Verification items for the finished model (mm, model axes). Give positions to 0.01 mm unless a question says otherwise; leave off trailing zeros. Order: outer loops, then holes, each group sorted by start corner. A loop starts at its lowest first (then second) coordinate and runs counter-clockwise, first axis right, second up. Notation, with made-up numbers: (-23, 75) -> (3, 75) arc R14 ccw to (3, 86) -> close; hole circle Ø10 at (-13, 23.5). An arc over 180 degrees is marked (long way). Return JSON: item names as keys, results as strings. Group by question number.
(1) Release check for a two-part mould opening along Y. For faces 1 (the face through (16.31, 40.067, 57.291)), 2 (the face through (18, 38, 0)), 3 (the face through (18.13, 46.87, 55.71)) record: pulls with the +Y half, pulls with the -Y half, needs draft (parallel to the pull), parting line crosses it, or undercut.
(2) Thickness scan on line 1 along Y through (x, z) = (16.25, 99); line 2 along Y through (x, z) = (18.5, 8); line 3 along X through (y, z) = (39.75, 71.5). Record the ranges inside material, lowest first.
(3) Cross-section at A-A on z = 100.5. Enter the section's corners in (x, y).
(4) Depth check by flat-ended pin: pin 1 Ø4 at (y, z) = (33.5, 20) entering from -X; pin 2 Ø1.5 at (y, z) = (42.5, 31) entering from -X; pin 3 Ø5 at (x, y) = (17.5, 40.98) entering from -Z; pin 4 Ø4 at (x, z) = (14, 77) entering from +Y. Enter the tip coordinate at first touch or a pass-through.
from build123d import *

# Parameters (mm, degrees)
RESSALTO_EXTRUS_O1_DEPTH = 113
ESBO_O2_R                = 1.5
CORTE_EXTRUS_O1_DEPTH    = 113


with BuildPart() as part:
    # Esboço1 → Ressalto-extrusão1 (new body)
    with BuildSketch(Plane.XY):
        Polygon((11.5, 30.979337094), (21.5, 30.979337094), (21.5, 49.687624028), (21.161059666, 49.456664041), (19.066345307, 47.808952584), (17.161004874, 45.902414631), (15.486453, 43.765993321), (14.074906639, 41.431162512), (12.967287062, 38.97151993), (12.155978451, 36.372733292), (11.660337074, 33.660653998), align=None)
    extrude(amount=RESSALTO_EXTRUS_O1_DEPTH)

    # Esboço2 → Corte-extrusão1 (cut)
    with BuildSketch(Plane.XY.offset(113)):
        with Locations((17.5, 34.979337094)):
            Circle(ESBO_O2_R)
        with Locations((17.5, 40.979337094)):
            Circle(ESBO_O2_R)
    extrude(amount=-CORTE_EXTRUS_O1_DEPTH, mode=Mode.SUBTRACT)


solid = part.part
Verdict:
{
 "1": {"face 1": "undercut", "face 2": "needs draft", "face 3": "pulls with the +Y half"},
 "2": {"line 1": "30.98 to 34.15, 35.81 to 40.15, 41.81 to 44.74", "line 2": "30.98 to 33.86, 36.1 to 39.86, 42.1 to 47.24", "line 3": "13.32 to 16.64, 18.36 to 21.5"},
 "3": {"outline": "(11.5, 30.98) -> (21.5, 30.98) -> (21.5, 49.69) -> (21.16, 49.46) -> (19.07, 47.81) -> (17.16, 45.9) -> (15.49, 43.77) -> (14.07, 41.43) -> (12.97, 38.97) -> (12.16, 36.37) -> (11.66, 33.66) -> close; hole circle Ø3 at (17.5, 34.98); hole circle Ø3 at (17.5, 40.98)"},
 "4": {"pin 1": "x = 11.53", "pin 2": "x = 14.27", "pin 3": "z = 0", "pin 4": "y = 44.42"}
}
